Part print with two shaded views. Sizes in mm from the minimum x, y, z corner. Give positions to 0.01 mm unless a question says otherwise; leave off trailing zeros. Order: outer loops, then holes, each group sorted by start corner. A loop starts at its lowest first (then second) coordinate and runs counter-clockwise, first axis right, second up. Notation, with made-up numbers: M -24,-5 L 17,-5 A23 cw 17,17 Z; hole C 89.5,-15.75 d8. An arc over 180 degrees is marked long. Answer as CSV lines item,"result".
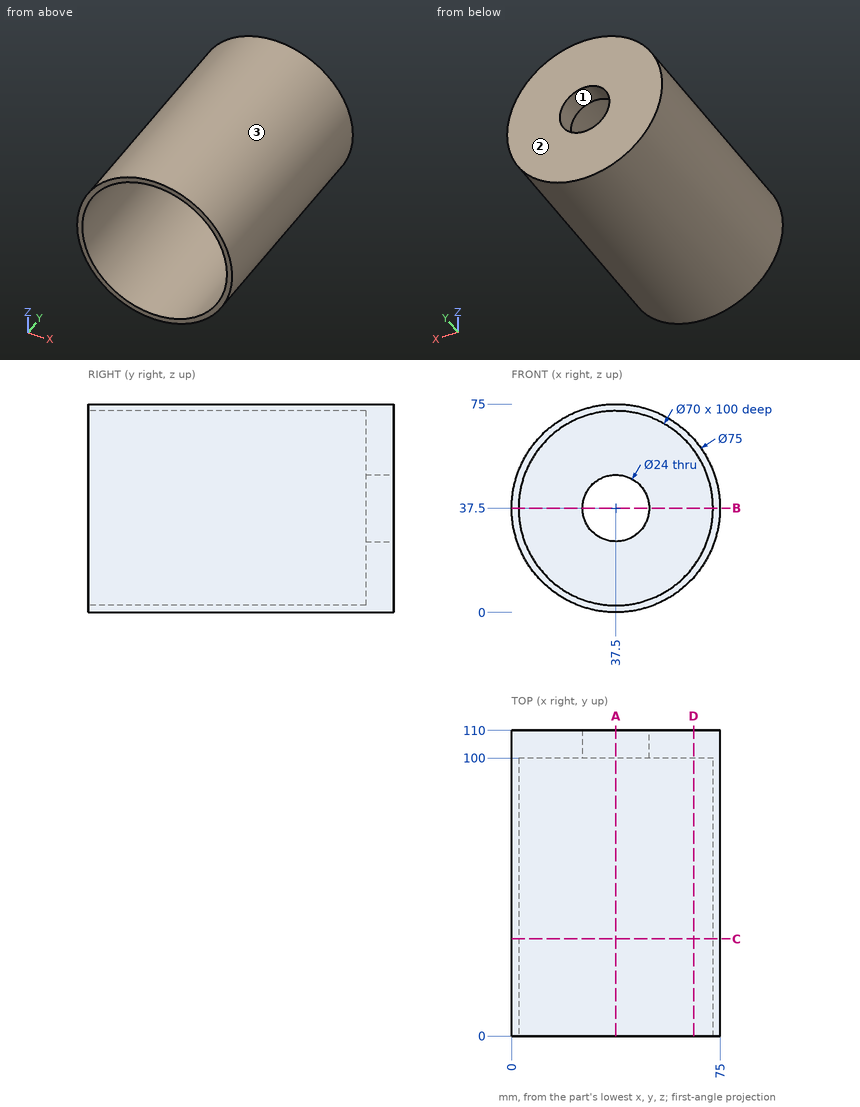
Item 1: Band-saw the part on B-B (z = 37.5). Give the cut face in (x, y).
Geometry says:
outline,"M 0,0 L 2.5,0 L 2.5,100 L 25.5,100 L 25.5,110 L 0,110 Z; M 49.5,100 L 72.5,100 L 72.5,0 L 75,0 L 75,110 L 49.5,110 Z"
Item 2: Band-saw the part on C-C (y = 35). Give the cut face in (x, z), and give its area (3 significant figures).
Geometry says:
outline,"C 37.5,37.5 d75; hole C 37.5,37.5 d70"
area,"569 mm2"
Item 3: Band-saw the part on D-D (x = 65.5). Give the cut face in (y, z), and give its area (3 significant figures).
Geometry says:
outline,"M 0,12.56 L 110,12.56 L 110,62.44 L 0,62.44 L 0,58.5 L 100,58.5 L 100,16.5 L 0,16.5 Z"
area,"1,290 mm2"
Item 4: Band-saw the part on A-A (x = 37.5). Give the cut face in (y, z), and give its area (3 significant figures).
Geometry says:
outline,"M 0,0 L 110,0 L 110,25.5 L 100,25.5 L 100,2.5 L 0,2.5 Z; M 0,72.5 L 100,72.5 L 100,49.5 L 110,49.5 L 110,75 L 0,75 Z"
area,"1,010 mm2"
Item 5: Pull direction Z, two halves, no side cores. Call the marked faces 1, 2 and 3: released by +Z, released by -Z, zero draft, split by the parting line, or undercut.
Geometry says:
face 1,"undercut"
face 2,"zero draft"
face 3,"split by the parting line"
Item 6: Probe line 1 along Y through (x, z) = (60, 30); line 2 along Z through (x, y) = (37, 103); line 3 along Z through (x, y) = (36, 8). List the from-to ranges inside material, lowest first. Write a range as from..to.
Geometry says:
line 1,"y = 100..110"
line 2,"z = 0..25.51, 49.49..75"
line 3,"z = 0.03..2.53, 72.47..74.97"
Item 7: Drop flat-ended pins along their axis: pin 1 (6 mm diameter, centred on x = 32, y = 60, fed in from +Z); pin 2 (21 mm diameter, centred on x = 30, z = 48, fed in from -Y); pin 3 (6 mm diameter, centred on x = 47, y = 71.5, fed in from +Z); pin 4 (21.5 mm diameter, centred on x = 37.5, z = 37.5, fed in from +Y). Give the stop position or say it passes through.
Geometry says:
pin 1,"stops at z = 74.92"
pin 2,"stops at y = 100"
pin 3,"stops at z = 74.43"
pin 4,"passes through"
